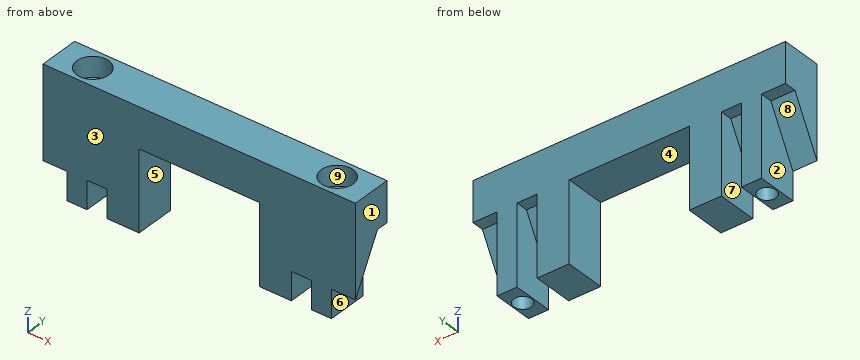
```python
from build123d import *

# Parameters (mm, degrees)
SKETCH_W        = 78
SKETCH_H        = 10
PAD_DEPTH       = 30
POCKET_DEPTH    = 5
POCKET001_DEPTH = 174.334003
SKETCH003_R     = 2.25
POCKET002_DEPTH = 198.334003
SKETCH004_R     = 4
POCKET003_DEPTH = 5
SKETCH005_W     = 30
SKETCH005_H     = 10
POCKET004_DEPTH = 20


with BuildPart() as part:
    # Sketch → Pad (new body)
    with BuildSketch(Plane.XY):
        Rectangle(SKETCH_W, SKETCH_H)
    extrude(amount=PAD_DEPTH)

    # Sketch001 (on DatumPlane) → Pocket (cut)
    with BuildSketch(Plane.YZ.offset(23)):
        Polygon((-5, 0), (5, 0), (5, 20), (2, 20), (-5, 7), align=None)
    pocket = extrude(amount=POCKET_DEPTH, mode=Mode.SUBTRACT)

    # Sketch002 (on DatumPlane) → Pocket001 (cut, through all)
    with BuildSketch(Plane.YZ.offset(33)):
        Polygon((-5, 0), (5, 0), (5, 20), (2, 20), (-5, 7), align=None)
    pocket001 = extrude(amount=POCKET001_DEPTH, mode=Mode.SUBTRACT)

    # Sketch003 (on Face5 of Pocket001) → Pocket002 (cut, through all)
    with BuildSketch(Plane.XY.offset(30)):
        with Locations((30.5, 0)):
            Circle(SKETCH003_R)
    pocket002 = extrude(amount=-POCKET002_DEPTH, mode=Mode.SUBTRACT)

    # Sketch004 (on Face5 of Pocket002) → Pocket003 (cut)
    with BuildSketch(Plane.XY.offset(30)):
        with Locations((30.5, 0)):
            Circle(SKETCH004_R)
    pocket003 = extrude(amount=-POCKET003_DEPTH, mode=Mode.SUBTRACT)

    # Mirrored: Pocket003, Pocket002, Pocket001, Pocket across YZ
    add(pocket003.mirror(Plane.YZ), mode=Mode.SUBTRACT)
    add(pocket002.mirror(Plane.YZ), mode=Mode.SUBTRACT)
    add(pocket001.mirror(Plane.YZ), mode=Mode.SUBTRACT)
    add(pocket.mirror(Plane.YZ), mode=Mode.SUBTRACT)

    # Sketch005 (on Face12 of Mirrored) → Pocket004 (cut)
    with BuildSketch(Plane(origin=(0, 0, 0), x_dir=(1, 0, 0), z_dir=(0, 0, -1))):
        Rectangle(SKETCH005_W, SKETCH005_H)
    extrude(amount=-POCKET004_DEPTH, mode=Mode.SUBTRACT)


solid = part.part
```
Model file for the job. Use its own axes, mm. Face numbers are marked on the shaded views. A direction names the side the tool comes from. Coordinates: 2 decimals unless noted, no trailing zeros. Loops run counter-clockwise (first coordinate to the right, second up) from the corner with the lowest first, then second, coordinate; pieces in that order, holes last. Notation, with made-up numbers: M -31,8.5 L 5,8.5 A9 cw 5,13.5 Z; hole C -28,-1 d2. An arc over 180 degrees is marked long. Use CSV: the item, a comma, the result in double quotes. Start each with the question number.
1. Band-saw the part on A-A, the plane x = -30.5. List the corners of the cut face in (y, z).
2. Band-saw the part on C-C, the plane z = 27.25. List the corners of the cut face in (x, y), then the cut area to 3 significant figures.
3. Band-saw the part on B-B, the plane z = 15. List the corners of the cut face in (x, y), then the cut area to 3 significant figures.
4. Tool access for the marked faces 5, 6, 7, 8 and 9: list every direction of +Z, -Z, +X, -X, +Y, -Y with a clear straight run to the whole face (end or side of a thin tool).
5. Band-saw the part on D-D, the plane y = 0. Give the number of separate pieces and of enclosed holes in the cut face, then the cut area to 3 significant figures.
6. Two-plate mould, pull along X, no slides. Class the marked faces 1, 2, 3 and 4: pulls with the +X half, pulls with the -X half, needs draft (parallel to the pull), parting line crosses it, or undercut.
7. Probe probe 1 along X at (y, z) = (-1.5, 25.5); probe 2 along X at (y, z) = (1.25, 5.25); probe 3 along Y at (x, z) = (30.5, 27). List the from-to ranges inside material, lowest first. Write a range as [from, to].
8. Flat gauge pins, fed straight in: pin 1 (5 mm diameter, centred on y = 2.5, z = 6.5, fed in from -X); pin 2 (1.5 mm diameter, centred on x = 24.5, y = 3.5, fed in from -Z); pin 3 (12 mm diameter, centred on x = 5, z = 15, fed in from -Y); pin 4 (3 mm diameter, centred on y = -2, z = 6.5, fed in from +X). Where does each tip first touch, or does it go through?
Entries:
1,outline,"M -5,0 L -2.25,0 L -2.25,25 L -4,25 L -4,30 L -5,30 Z; M 2.25,0 L 5,0 L 5,30 L 4,30 L 4,25 L 2.25,25 Z"
2,outline,"M -39,-5 L 39,-5 L 39,5 L -39,5 Z; hole C -30.5,0 d8; hole C 30.5,0 d8"
2,area,"679 mm2"
3,outline,"M -39,-5 L -15,-5 L -15,5 L -23,5 L -23,-0.69 L -28,-0.69 L -28,5 L -33,5 L -33,-0.69 L -39,-0.69 Z; M 15,-5 L 39,-5 L 39,-0.69 L 33,-0.69 L 33,5 L 28,5 L 28,-0.69 L 23,-0.69 L 23,5 L 15,5 Z; hole C -30.5,0 d4.5; hole C 30.5,0 d4.5"
3,area,"323 mm2"
4,face 5,"-Z, +Y, -Y"
4,face 6,"-Z, +X, +Y"
4,face 7,"-Z, +Y"
4,face 8,"-Z, -X, +Y"
4,face 9,"+Z"
5,separate pieces,"3"
5,enclosed holes,"0"
5,area,"1,080 mm2"
6,face 1,"pulls with the +X half"
6,face 2,"pulls with the -X half"
6,face 3,"needs draft"
6,face 4,"undercut"
7,probe 1,"x = [-39, -34.21], [-26.79, 26.79], [34.21, 39]"
7,probe 2,"x = [-33, -32.37], [-28.63, -28], [-23, -15], [15, 23], [28, 28.63], [32.37, 33]"
7,probe 3,"y = [-5, -4], [4, 5]"
8,pin 1,"stops at x = -33"
8,pin 2,"stops at z = 20"
8,pin 3,"stops at y = -5"
8,pin 4,"stops at x = 33"
